```python
from build123d import *

# Parameters (mm, degrees)
SKETCH1_W           = 50
SKETCH1_H           = 53.3
BOSS_EXTRUDE1_DEPTH = 3.175
SKETCH2_W           = 50
SKETCH2_H           = 3
BOSS_EXTRUDE2_DEPTH = 48.97
SKETCH3_W           = 3.175
SKETCH3_H           = 15
SKETCH3_H_2         = 15.175
BOSS_EXTRUDE3_DEPTH = 20
CUT_EXTRUDE1_DEPTH  = 65
SKETCH5_R           = 11
SKETCH5_R_2         = 1.7
CUT_EXTRUDE2_DEPTH  = 65
CUT_EXTRUDE3_DEPTH  = 65
CHAMFER1_SIZE       = 5
FILLET1_R           = 5


with BuildPart() as part:
    # Sketch1 → Boss-Extrude1 (new body)
    with BuildSketch(Plane(origin=(0, 0, 0), x_dir=(1, 0, 0), z_dir=(0, 1, 0))):
        with Locations((25, 26.65)):
            Rectangle(SKETCH1_W, SKETCH1_H)
    extrude(amount=BOSS_EXTRUDE1_DEPTH)

    # Sketch2 → Boss-Extrude2 (add)
    with BuildSketch(Plane(origin=(0, 3.175, 0), x_dir=(1, 0, 0), z_dir=(0, 1, 0))):
        with Locations((25, 1.5)):
            Rectangle(SKETCH2_W, SKETCH2_H)
    extrude(amount=BOSS_EXTRUDE2_DEPTH)

    # Sketch3 → Boss-Extrude3 (add)
    with BuildSketch(Plane(origin=(0, 3.175, 0), x_dir=(1, 0, 0), z_dir=(0, 1, 0))):
        with Locations((1.5875, 10.5)):
            Rectangle(SKETCH3_W, SKETCH3_H)
        with Locations((48.4125, 10.5875)):
            Rectangle(SKETCH3_W, SKETCH3_H_2)
    extrude(amount=BOSS_EXTRUDE3_DEPTH)

    # Sketch4 → Cut-Extrude1 (cut)
    with BuildSketch(Plane(origin=(50, 0, 0), x_dir=(0, 0, -1), z_dir=(1, 0, 0))):
        Polygon((18.175, 3.175), (3, 23.175), (18.175, 23.175), align=None)
    extrude(amount=-CUT_EXTRUDE1_DEPTH, mode=Mode.SUBTRACT)

    # Sketch5 → Cut-Extrude2 (cut)
    with BuildSketch(Plane.XY):
        with Locations((25, 31.145)):
            Circle(SKETCH5_R)
        with Locations((40.502, 46.647)):
            Circle(SKETCH5_R_2)
        with Locations((9.528, 46.677)):
            Circle(SKETCH5_R_2)
        with Locations((9.498, 15.703)):
            Circle(SKETCH5_R_2)
        with Locations((40.472, 15.673)):
            Circle(SKETCH5_R_2)
    extrude(amount=-CUT_EXTRUDE2_DEPTH, mode=Mode.SUBTRACT)

    # Sketch6 → Cut-Extrude3 (cut)
    with BuildSketch(Plane(origin=(0, 3.175, 0), x_dir=(1, 0, 0), z_dir=(0, 1, 0))):
        with BuildLine():
            ThreePointArc((42.125, 42.3), (40, 44.425), (37.875, 42.3))
            Line((37.875, 42.3), (37.875, 12.3))
            ThreePointArc((37.875, 12.3), (40, 10.175), (42.125, 12.3))
            Line((42.125, 12.3), (42.125, 42.3))
        make_face()
        with BuildLine():
            Line((7.875, 42.3), (7.875, 12.3))
            ThreePointArc((7.875, 12.3), (10, 10.175), (12.125, 12.3))
            Line((12.125, 12.3), (12.125, 42.3))
            ThreePointArc((12.125, 42.3), (10, 44.425), (7.875, 42.3))
        make_face()
    extrude(amount=-CUT_EXTRUDE3_DEPTH, mode=Mode.SUBTRACT)

    # Chamfer1
    chamfer1_edges = [part.edges().sort_by_distance(p)[0] for p in [
        (0, 1.5875, -53.3),
        (50, 1.5875, -53.3),
        (0, 52.145, -1.5),
        (50, 52.145, -1.5),
    ]]
    chamfer(chamfer1_edges, length=CHAMFER1_SIZE)

    # Fillet1
    fillet1_edges = [part.edges().sort_by_distance(p)[0] for p in [
        (25, 3.175, -3),
        (25, 0, 0),
    ]]
    fillet(fillet1_edges, radius=FILLET1_R)


solid = part.part
```
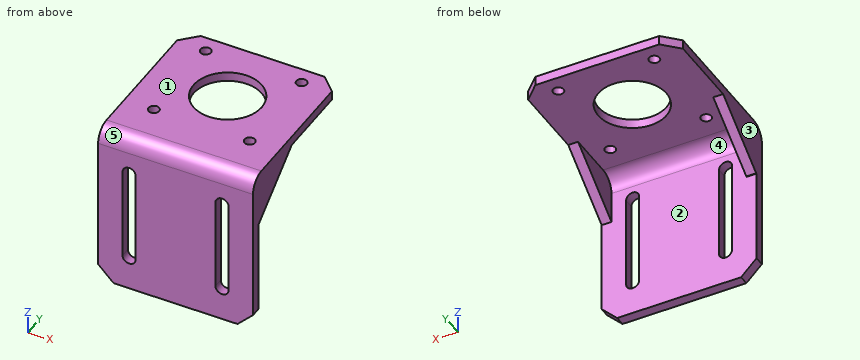
Source: CAD feature listing. Evaluate the final solid. Frame: model axes, mm. Face numbers are marked on the shaded views. A direction names the side the tool comes from. Round coordinates to 2 decimals unless told otherwise and drop trailing zeros. Loops run counter-clockwise (first coordinate to the right, second up) from the corner with the lowest first, then second, coordinate; pieces in that order, holes last. Notation, with made-up numbers: M -13,-16 L 8,-16 A14 cw 8,-12 Z; hole C -10,-37.75 d11. An arc over 180 degrees is marked long. Put each result on its own line as item: value.
(1) Section B-B, the plane x = 40. Return loops of the section in (y, z) (3 decimals).
Solutions:
outline: M 0,-53.3 L 3.175,-53.3 L 3.175,-44.425 L 0,-44.425 Z; M 0,-10.175 L 3.175,-10.175 L 3.175,-8 A5 cw 8.175,-3 L 14.04,-3 L 14.04,0 L 5,0 A5 ccw 0,-5 Z; M 17.306,-3 L 45.023,-3 L 45.023,0 L 17.306,0 Z; M 48.271,-3 L 52.145,-3 L 52.145,0 L 48.271,0 Z
(2) Ray query, line 1 (X direction, y = 3, z = -31) (3 decimals); line 2 (Z direction, x = 39, y = 9); line 3 (Y direction, x = 25.5, z = -34) (3 decimals). Return the intervals inside material, ascending. Write a range as [from, to].
Solutions:
line 1: [0, 7.875], [12.125, 37.875], [42.125, 50]
line 2: [-3, 0]
line 3: [0, 3.175]
(3) Section A-A, the plane z = -24.5. Return loops of the section in (x, y) (3 decimals).
Solutions:
outline: M 0,0 L 7.875,0 L 7.875,3.175 L 0,3.175 Z; M 12.125,0 L 37.875,0 L 37.875,3.175 L 12.125,3.175 Z; M 42.125,0 L 50,0 L 50,3.175 L 42.125,3.175 Z
(4) Section D-D, the plane x = 28.5. Return loops of the section in (y, z) (3 decimals).
Solutions:
outline: M 0,-53.3 L 3.175,-53.3 L 3.175,-8 A5 cw 8.175,-3 L 20.717,-3 L 20.717,0 L 5,0 A5 ccw 0,-5 Z; M 41.573,-3 L 52.145,-3 L 52.145,0 L 41.573,0 Z
(5) Access query for the marked faces 4 and 5. Directions: +Z, -Z, +X, -X, +Y, -Y. A direction counts if a zero-diameter tool reaches every point of the face in a straight line with its end or side. Return the directions, or none.
Solutions:
face 4: -Z, +Y
face 5: +Z, +X, -X, -Y
(6) First-contact query: pin 1 (8 mm diameter, centred on x = 13, y = 33, fed in from -Z); pin 2 (10 mm diameter, centred on x = 21.5, z = -47.5, fed in from -Y); pin 3 (1.5 mm diameter, centred on x = 11, y = 7, fed in from -Z); pin 4 (13.5 mm diameter, centred on x = 15, z = -24, fed in from +Y) (3 decimals). Flat tips, straight axial feed; report the tip coordinate or a pass-through.
Solutions:
pin 1: z = -3
pin 2: y = 0
pin 3: z = -3.39
pin 4: y = 3.175
(7) Pull-direction query (X, two-part tool) for the marked faces 1, 2 and 3; classes: released by +X, released by -X, zero draft, split by the parting line, or undercut.
Solutions:
face 1: zero draft
face 2: undercut
face 3: released by -X
(8) Section C-C, the plane y = 36.5. Return loops of the section in (x, z), and give its area (3 significant figures).
Solutions:
outline: M 0,-3 L 15.39,-3 L 15.39,0 L 0,0 Z; M 34.61,-3 L 50,-3 L 50,0 L 34.61,0 Z
area: 92.3 mm²
